from build123d import *

# Parameters (mm, degrees)
SKETCH1_W              = 88.9
SKETCH1_H              = 50.8
SKETCH1_R              = 15.875
BOSS_EXTRUDE1_DEPTH    = 1.5875
F_10_CLEARANCE_HOLE1_D = 5.6134


with BuildPart() as part:
    # Sketch1 → Boss-Extrude1 (new body)
    with BuildSketch(Plane.XY):
        with Locations((25.49525, 0)):
            Rectangle(SKETCH1_W, SKETCH1_H)
        Circle(SKETCH1_R, mode=Mode.SUBTRACT)
        with Locations((50.9905, 0)):
            Circle(SKETCH1_R, mode=Mode.SUBTRACT)
    extrude(amount=BOSS_EXTRUDE1_DEPTH)

    # #10 Clearance Hole1 (through all)
    with Locations(Plane(origin=(-41.275, -44.45, 1.5875), x_dir=(1, 0, 0), z_dir=(0, 0, 1))):
        with Locations((104.87025, 63.5), (28.67025, 63.5), (66.77025, 25.4), (28.67025, 25.4), (66.77025, 63.5), (104.87025, 25.4)):
            Hole(F_10_CLEARANCE_HOLE1_D / 2)


solid = part.part
Verification items for the finished model (mm, model axes). Give positions to 0.01 mm unless a question says otherwise; leave off trailing zeros. Order: outer loops, then holes, each group sorted by start corner. A loop starts at its lowest first (then second) coordinate and runs counter-clockwise, first axis right, second up. Notation, with made-up numbers: (84, 44) -> (123, 44) arc R12 cw to (123, 48) -> close; hole circle Ø11 at (-6.75, 35). An arc over 180 degrees is marked (long way). Answer as CSV lines item,"result".
Q1. Release check for a two-part mould opening along Y. For faces 1 (the flat face through (25, -25.4, 1)), 2 (the cylindrical face through (65.655, -6.08, 0.783)), 3 (the flat face through (69.945, 0, 1)), 4 (the flat face through (25, 25.4, 1)) record: +Y half, -Y half, draft (parallel to the pull), parting line (faces both ways), or undercut.
Solutions:
face 1,"-Y half"
face 2,"undercut"
face 3,"draft"
face 4,"+Y half"
Q2. Sectioned sample at B-B on x = 0. Record the cut outline in (y, z) (1 decimal), plus the area to 3 significant figures.
Solutions:
outline,"(-25.4, 0) -> (-15.9, 0) -> (-15.9, 1.6) -> (-25.4, 1.6) -> close; (15.9, 0) -> (25.4, 0) -> (25.4, 1.6) -> (15.9, 1.6) -> close"
area,"30.2 mm²"
Q3. Sectioned sample at D-D on y = 0. Record the cut outline in (x, z) (1 decimal).
Solutions:
outline,"(-19, 0) -> (-15.9, 0) -> (-15.9, 1.6) -> (-19, 1.6) -> close; (15.9, 0) -> (35.1, 0) -> (35.1, 1.6) -> (15.9, 1.6) -> close; (66.9, 0) -> (69.9, 0) -> (69.9, 1.6) -> (66.9, 1.6) -> close"
Q4. Sectioned sample at C-C on z = 1.05. Count the separate pieces of the cut face and the enclosed holes in it, plus the area to 3 significant figures.
Solutions:
separate pieces,"1"
enclosed holes,"8"
area,"2,780 mm²"
Q5. Scan lines: probe 1 along X at (y, z) = (5.5, 0.4); probe 2 along Y at (x, z) = (0, 1.25) (3 decimals); probe 3 along X at (y, z) = (-2.5, 1.2). Record each from-to range of solid material in increasing order.
Solutions:
probe 1,"x = -18.95 to -14.89, 14.89 to 36.1, 65.88 to 69.95"
probe 2,"y = -25.4 to -15.875, 15.875 to 25.4"
probe 3,"x = -18.95 to -15.68, 15.68 to 35.31, 66.67 to 69.95"
Q6. Sectioned sample at A-A on y = 19.05. Record the cut outline in (x, z).
Solutions:
outline,"(-18.95, 0) -> (-15.41, 0) -> (-15.41, 1.59) -> (-18.95, 1.59) -> close; (-9.8, 0) -> (22.69, 0) -> (22.69, 1.59) -> (-9.8, 1.59) -> close; (28.3, 0) -> (60.79, 0) -> (60.79, 1.59) -> (28.3, 1.59) -> close; (66.4, 0) -> (69.95, 0) -> (69.95, 1.59) -> (66.4, 1.59) -> close"
